```python
from build123d import *

# Parameters (mm, degrees)
SKETCH1_R           = 5
BOSS_EXTRUDE1_DEPTH = 5
SKETCH2_R           = 4.9
BOSS_EXTRUDE2_DEPTH = 10
BOSS_EXTRUDE3_START = -1
SKETCH4_R           = 5
BOSS_EXTRUDE3_DEPTH = 1


with BuildPart() as part:
    # Sketch1 → Boss-Extrude1 (new body)
    with BuildSketch(Plane(origin=(0, 0, 0), x_dir=(1, 0, 0), z_dir=(0, 1, 0))):
        with BuildLine():
            Line((0, 0), (15, 0))
            ThreePointArc((15, 0), (22.5, 7.5), (15, 15))
            Line((15, 15), (0, 15))
            ThreePointArc((0, 15), (-7.5, 7.5), (0, 0))
        make_face()
        with Locations(Location((15, 7.5, 0), (0, 0, 270))):
            Circle(SKETCH1_R, mode=Mode.SUBTRACT)
        with BuildLine():
            Line((4.582575695, 5.5), (2.082575695, 5.5))
            Line((2.082575695, 5.5), (2.082575695, 9.5))
            Line((2.082575695, 9.5), (4.582575695, 9.5))
            ThreePointArc((4.582575695, 9.5), (-5, 7.5), (4.582575695, 5.5))
        make_face(mode=Mode.SUBTRACT)
    extrude(amount=BOSS_EXTRUDE1_DEPTH)



with BuildPart() as body_2:
    # Sketch2 → Boss-Extrude2 (new body)
    with BuildSketch(Plane(origin=(0, 5, 0), x_dir=(1, 0, 0), z_dir=(0, 1, 0))):
        with Locations(Location((15, 7.5, 0), (0, 0, 270))):
            Circle(SKETCH2_R)
    extrude(amount=-BOSS_EXTRUDE2_DEPTH)


with BuildPart() as part_1:
    add(part.part)

    add(body_2.part)  # Boss-Extrude3 merges body 2
    # Sketch4 → Boss-Extrude3 (add)
    with BuildSketch(Plane(origin=(0, 5, 0), x_dir=(-1, 0, 0), z_dir=(0, 1, 0)).offset(BOSS_EXTRUDE3_START)):
        with Locations(Location((-15, -7.5, 0), (0, 0, 90))):
            Circle(SKETCH4_R)
    extrude(amount=BOSS_EXTRUDE3_DEPTH)


solid = part_1.part
```
Input: part model. Units: mm. Frame: model coordinates. A direction names the side the tool comes from. Coordinates: 2 decimals unless noted, no trailing zeros. Write each loop counter-clockwise with the first axis right and the second up, starting at its lowest first coordinate (ties: lowest second). Pieces come first, ordered by that corner, then holes. Notation, with made-up numbers: (-31, 0.5) -> (20, 0.5) arc R27 ccw to (20, 30.5) -> close; hole circle Ø1 at (-0.5, 26). An arc over 180 degrees is marked (long way). Answer as a JSON object with one key per item and string values.
1. Material intervals for line 1 (Z direction, x = 3.25, y = 3.25); line 2 (Z direction, x = 0, y = 2.9); line 3 (Y direction, x = 4.25, z = -3.5), sorted ascending. Write a range as from..to.
Result set:
{"line 1": "z = -15..-11.3, -9.5..-5.5, -3.7..0", "line 2": "z = -15..-12.5, -2.5..0", "line 3": "y = 0..5"}
2. Section D-D on x = 18.25. Return the cut outline in (y, z), then the cut area to 3 significant figures.
Result set:
{"outline": "(-5, -11.17) -> (4, -11.17) -> (4, -11.3) -> (0, -11.3) -> (0, -14.26) -> (5, -14.26) -> (5, -0.74) -> (0, -0.74) -> (0, -3.7) -> (4, -3.7) -> (4, -3.83) -> (-5, -3.83) -> close", "area": "103 mm2"}
3. Mould query, pull axis X, two halves, no side actions, for faces 3 (the face through (13.123, -0.437, -2.974)), 4 (the face through (-4.996, 2.465, -7.691)), 5 (the face through (22.5, 2.46, -7.34)), 6 (the face through (7, 0, -8)). Classes: released by +X, released by -X, zero draft, split by the parting line, or undercut.
Result set:
{"face 3": "undercut", "face 4": "undercut", "face 5": "released by +X", "face 6": "zero draft"}
4. Section C-C on x = -2. Return the cut outline in (y, z), then the cut area to 3 significant figures.
Result set:
{"outline": "(0, -14.73) -> (5, -14.73) -> (5, -12.08) -> (0, -12.08) -> close; (0, -2.92) -> (5, -2.92) -> (5, -0.27) -> (0, -0.27) -> close", "area": "26.5 mm2"}
5. Access query for faces 1 (the face through (3, 2, -5.5)), 2 (the face through (8, 2, -15)). Directions: +Z, -Z, +X, -X, +Y, -Y. A direction counts if a zero-diameter tool reaches every point of the face in a straight line with its end or side. Return the directions, or none.
Result set:
{"face 1": "+Y, -Y", "face 2": "-Z, +X, -X, +Y, -Y"}
6. First-contact query: P1, Ø2, axis at x = 17, y = 1, coming from the -Z side; P2, Ø2, axis at x = -2.5, y = 0, coming from the +Z side; P3, Ø3, axis at y = -2.5, z = -8.5, coming from the -X side. Flat tips, straight axial feed; report the tip coordinate or a pass-through.
Result set:
{"P1": "stops at z = -14.93", "P2": "stops at z = -0.15", "P3": "stops at x = 10.1"}
7. Section B-B on z = -7.5. Return the cut outline in (x, y).
Result set:
{"outline": "(-7.5, 0) -> (-5, 0) -> (-5, 5) -> (-7.5, 5) -> close; (2.08, 0) -> (10, 0) -> (10, 4) -> (10.1, 4) -> (10.1, -5) -> (19.9, -5) -> (19.9, 4) -> (20, 4) -> (20, 0) -> (22.5, 0) -> (22.5, 5) -> (2.08, 5) -> close"}
8. Section A-A on y = 1.5. Return the cut outline in (x, z), then the cut area to 3 significant figures.
Result set:
{"outline": "(0, -15) -> (15, -15) arc R7.5 ccw to (15, 0) -> (0, 0) arc R7.5 ccw to start; circle Ø9.8 at (15, -7.5); hole (2.08, -9.5) -> (2.08, -5.5) -> (4.58, -5.5) arc R5 ccw (long way) to (4.58, -9.5) -> close; hole circle Ø10 at (15, -7.5)", "area": "331 mm2"}
